For this review, take the finished solid that the model builds, in its own axes (mm). Coordinates: 2 decimals unless noted, no trailing zeros. Order: outer loops, then holes, each group sorted by start corner. A loop starts at its lowest first (then second) coordinate and runs counter-clockwise, first axis right, second up. Notation, with made-up numbers: (14.5, 85) -> (69.5, 85) arc R16 cw to (69.5, 111) -> close; hole circle Ø7 at (19.5, 69.25). An arc over 180 degrees is marked (long way). Return JSON: item names as keys, results as strings. Group by question number.
Item 1: Take a section at B-B (x = 46). Write out the cut boundary in (y, z).
Item 2: Take a section at A-A (y = -36). Write out the cut boundary in (x, z).
Item 3: Draft analysis for pull direction Y (two halves, no side actions). For faces 1 (the flat face through (-1, 1, 3)), 2 (the flat face through (1, -40, 1)), 3 (the cylindrical face through (-44.536, 36.325, 1.479)), 4 (the cylindrical face through (47.464, 36.325, 1.479)), state which applies: +Y half, -Y half, draft (parallel to the pull), parting line (faces both ways), or undercut.
Item 4: For line 1 along Y through (x, z) = (46, 1.6); line 2 along X through (y, z) = (-36, 2.05); line 3 along X through (y, z) = (37, 0.25), list the stretches that pass through material, from the lowest coordinate up.
Autodesk Inventor part; units mm, degrees
ref_plane "YZ Plane" through (0, 0, 0) normal (1, 0, 0) x (0, 1, 0)
ref_plane "XZ Plane" through (0, 0, 0) normal (0, 1, 0) x (-1, 0, 0)
ref_plane "XY Plane" through (0, 0, 0) normal (0, 0, 1) x (1, 0, 0)
sketch "スケッチ1" plane through (0, 0, 0) normal (0, 0, 1) x (1, 0, 0)
  line L0 (-50, 40) -> (50, 40)
  line L1 (50, 40) -> (50, -40)
  line L2 (50, -40) -> (-50, -40)
  line L3 (-50, -40) -> (-50, 40)
  line L4 (-50, 40) -> (50, -40) construction
  line L5 (50, 40) -> (-50, -40) construction
  point P0 (0, 0)
  dimension "d0" = 100
  dimension "d1" = 80
extrude "押し出し1" add sketch "スケッチ1" along normal blind 3
sketch "スケッチ2" plane through (0, 0, 3) normal (0, 0, 1) x (1, 0, 0)
  line L0 (-50, 40) -> (-50, -40)
  line L1 (50, 40) -> (-50, 40)
  line L2 (50, -40) -> (50, 40)
  line L3 (-50, -40) -> (50, -40)
  point P0 (0, 0)
  point P1 (-46, 36)
  point P2 (-46, -36)
  point P3 (46, -36)
  point P4 (46, -36)
  point P5 (46, 36)
  dimension "d4" = 4
  dimension "d5" = 4
  dimension "d6" = 4
  dimension "d7" = 4
hole "穴1" at (-46, 36, 3) at (-46, -36, 3) at (46, -36, 3) at (46, 36, 3) direction (0, 0, -1) diameter 3 end through all
properties part number "Main board ver2"
Findings below:
{
 "1": {"outline": "(-40, 0) -> (-37.5, 0) -> (-37.5, 3) -> (-40, 3) -> close; (-34.5, 0) -> (34.5, 0) -> (34.5, 3) -> (-34.5, 3) -> close; (37.5, 0) -> (40, 0) -> (40, 3) -> (37.5, 3) -> close"},
 "2": {"outline": "(-50, 0) -> (-47.5, 0) -> (-47.5, 3) -> (-50, 3) -> close; (-44.5, 0) -> (44.5, 0) -> (44.5, 3) -> (-44.5, 3) -> close; (47.5, 0) -> (50, 0) -> (50, 3) -> (47.5, 3) -> close"},
 "3": {"face 1": "draft", "face 2": "-Y half", "face 3": "undercut", "face 4": "undercut"},
 "4": {"line 1": "y = -40 to -37.5, -34.5 to 34.5, 37.5 to 40", "line 2": "x = -50 to -47.5, -44.5 to 44.5, 47.5 to 50", "line 3": "x = -50 to -47.12, -44.88 to 44.88, 47.12 to 50"}
}
